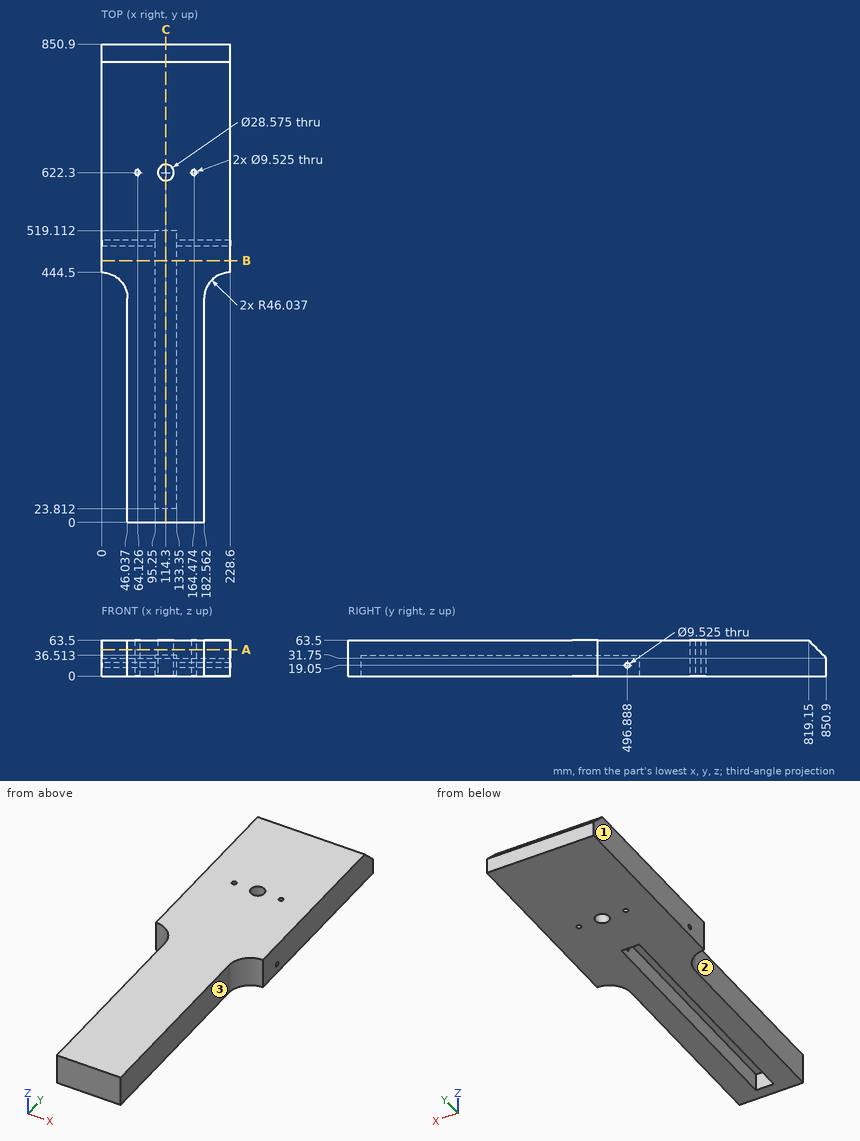
Design review of the part shown in the three views and the two pictorial views. Dimensions are in mm from the part's minimum x, y and z. A direction names the side the tool comes from. Give positions to 0.01 mm unless a question says otherwise; leave off trailing zeros. Write each loop counter-clockwise with the first axis right and the second up, starting at its lowest first coordinate (ties: lowest second). Pieces come first, ordered by that corner, then holes. Notation, with made-up numbers: (46.25, -4) -> (61.25, -4) arc R33 ccw to (61.25, 26) -> close; hole circle Ø6 at (61.5, 52.25). An arc over 180 degrees is marked (long way). Answer in a Markdown table with one row per item.
1) For L1, parallel to X at y = 622, z = 49 (1 decimal); L2, parallel to X at y = 368.5, z = 19; L3, parallel to X at y = 516, z = 20, list the stretches that pass through material, from the lowest coordinate up. Write a range as [from, to].
Worked answers:
| item | result |
|---|---|
| L1 | [0, 59.4], [68.9, 100], [128.6, 159.7], [169.2, 228.6] |
| L2 | [46.04, 95.25], [133.35, 182.56] |
| L3 | [0, 95.25], [133.35, 228.6] |
2) Clearance check with flat-ended pins moving along their axes: P1, Ø11, axis at x = 64.13, y = 622.3, coming from the +Z side; P2, Ø3, axis at x = 108, y = 320, coming from the -Z side; P3, Ø6, axis at x = 142, z = 48, coming from the +Y side; P4, Ø11, axis at y = 208.5, z = 25, coming from the -X side. State where each tip first meets the part, or that it passes through.
Worked answers:
| item | result |
|---|---|
| P1 | z = 63.5 |
| P2 | z = 36.51 |
| P3 | y = 837.65 |
| P4 | x = 46.04 |
3) Tool access review of the marked faces 1, 2 and 3: name each direction out of +Z, -Z, +X, -X, +Y, -Y from which nothing blocks a thin tool from reaching the whole face with its end or side.
Worked answers:
| item | result |
|---|---|
| face 1 | +Z, -Z, -X, +Y, -Y |
| face 2 | +Z, -Z, -X, -Y |
| face 3 | +Z, -Z, +X, -Y |
4) Add section B-B on y = 465.5. State the section outline as (x, z) points, plus the area to 3 significant figures.
Worked answers:
| item | result |
|---|---|
| outline | (0, 0) -> (95.25, 0) -> (95.25, 36.51) -> (133.35, 36.51) -> (133.35, 0) -> (228.6, 0) -> (228.6, 63.5) -> (0, 63.5) -> close |
| area | 13,100 mm² |
5) Add section A-A on z = 47. Count the separate pieces of the cut face and the enclosed holes in it, plus the area to 3 significant figures.
Worked answers:
| item | result |
|---|---|
| separate pieces | 1 |
| enclosed holes | 3 |
| area | 150,000 mm² |
6) Add section C-C on x = 114.3. State the section outline as (y, z) points, plus the area to 3 significant figures.
Worked answers:
| item | result |
|---|---|
| outline | (0, 0) -> (23.81, 0) -> (23.81, 36.51) -> (519.11, 36.51) -> (519.11, 0) -> (608.01, 0) -> (608.01, 63.5) -> (0, 63.5) -> close; (636.59, 0) -> (850.9, 0) -> (850.9, 31.75) -> (819.15, 63.5) -> (636.59, 63.5) -> close |
| area | 33,600 mm² |
